from build123d import *

# Parameters (mm, degrees)
SKETCH_1_W          = 71.7
SKETCH_1_H          = 30.5
EXTRUDE_1_DEPTH     = 25
SHELL_1_T           = -3
CUT_EXTRUDE_1_REACH = 48.29
SKETCH_2_W          = 30
SKETCH_2_H          = 10
SKETCH_3_W          = 9
SKETCH_3_H          = 9
EXTRUDE_2_DEPTH     = 10
SKETCH_4_R          = 4.924428901
CUT_EXTRUDE_2_DEPTH = 72.41207881
FILLET_1_R          = 0.2
EXTRUDE_3_DEPTH     = 9
FILLET_2_R          = 0.2
FILLET_3_R          = 0.5
MIRROR_START        = 15.5
MIRROR_2_DEPTH      = 9
FILLET_5_R          = 0.5
FILLET_6_R          = 0.5


# Read off the part's stored shape, not the designer's step: 镜向2
with BuildPart() as part:
    # 草图1 → 凸台-拉伸1 (new body)
    with BuildSketch(Plane.XY):
        Rectangle(SKETCH_1_W, SKETCH_1_H)
    extrude(amount=EXTRUDE_1_DEPTH)

    # 抽壳1
    shell_1_openings = [part.faces().sort_by_distance(p)[0] for p in [
        (35.85, 0, 12.5),
    ]]
    offset(amount=SHELL_1_T, openings=shell_1_openings, kind=Kind.INTERSECTION)

    # 草图2 → 切除-拉伸1 (cut, up to next)
    with BuildSketch(Plane(origin=(0, 0, 0), x_dir=(-1, 0, 0), z_dir=(0, 0, -1)), mode=Mode.PRIVATE) as cut_extrude_1_sk1:
        with Locations((17.35, -6.95)):
            Rectangle(SKETCH_2_W, SKETCH_2_H)
    cut_extrude_1_tool1 = extrude(cut_extrude_1_sk1.sketch, amount=-CUT_EXTRUDE_1_REACH, mode=Mode.PRIVATE) & part.part
    add(cut_extrude_1_tool1.solids().sort_by_distance((-17.35, -6.95, 0))[0], mode=Mode.SUBTRACT)

    # 草图3 → 凸台-拉伸2 (add)
    with BuildSketch(Plane.XY.offset(25)):
        with Locations((-20, 0)):
            Rectangle(SKETCH_3_W, SKETCH_3_H)
        with Locations((20, 0)):
            Rectangle(SKETCH_3_W, SKETCH_3_H)
    extrude(amount=EXTRUDE_2_DEPTH)

    # 草图4 → 切除-拉伸2 (cut, through all)
    with BuildSketch(Plane.ZY.offset(24.5)):
        with Locations((37, 0)):
            Circle(SKETCH_4_R)
    extrude(amount=-CUT_EXTRUDE_2_DEPTH, mode=Mode.SUBTRACT)

    # 圆角1
    fillet_1_edges = [part.edges().sort_by_distance(p)[0] for p in [
        (-20, 4.5, 35),
        (-20, -4.5, 35),
        (20, 4.5, 35),
        (20, -4.5, 35),
    ]]
    fillet(fillet_1_edges, radius=FILLET_1_R)

    # 草图5 → 凸台-拉伸3 (add)
    with BuildSketch(Plane.ZY.offset(24.5)):
        Polygon((34.212569003, 4.5), (32.769193331, 7), (30.446869021, 7), (30.446869021, 6), (32.191843061, 6), (33.057868465, 4.5), align=None)
        Polygon((32.769193331, -7), (30.446869021, -7), (30.446869021, -6), (32.191843061, -6), (33.057868465, -4.5), (34.212569003, -4.5), align=None)
    extrude(amount=-EXTRUDE_3_DEPTH)

    # 圆角2
    fillet_2_edges = [part.edges().sort_by_distance(p)[0] for p in [
        (-20, 6, 32.191843061),
        (-20, 6, 30.446869021),
        (-20, 7, 30.446869021),
        (-20, 7, 32.769193331),
        (-20, -7, 32.769193331),
        (-20, -7, 30.446869021),
        (-20, -6, 30.446869021),
        (-20, -6, 32.191843061),
    ]]
    fillet(fillet_2_edges, radius=FILLET_2_R)

    # 圆角3
    fillet_3_edges = [part.edges().sort_by_distance(p)[0] for p in [
        (-20, 4.5, 33.057868465),
        (-20, -4.5, 33.057868465),
    ]]
    fillet(fillet_3_edges, radius=FILLET_3_R)

    # 镜向2 outline → 镜向2 (add)
    with BuildSketch(Plane.YZ.offset(MIRROR_START)):
        with BuildLine():
            Line((5.25, 32.624855763), (5.9, 32.249578088))
            ThreePointArc((5.9, 32.249578088), (5.973205081, 32.176373007), (6, 32.076373007))
            Line((6, 32.076373007), (6, 30.646869021))
            ThreePointArc((6, 30.646869021), (6.058578644, 30.505447665), (6.2, 30.446869021))
            Line((6.2, 30.446869021), (6.8, 30.446869021))
            ThreePointArc((6.8, 30.446869021), (6.941421356, 30.505447665), (7, 30.646869021))
            Line((7, 30.646869021), (7, 32.653723277))
            ThreePointArc((7, 32.653723277), (6.973205081, 32.753723277), (6.9, 32.826928357))
            Line((6.9, 32.826928357), (4.5, 34.212569003))
            Line((4.5, 34.212569003), (4.5, 32.191843061))
            ThreePointArc((4.5, 32.191843061), (4.75, 32.624855763), (5.25, 32.624855763))
        make_face()
        with BuildLine():
            Line((-6.8, 30.446869021), (-6.2, 30.446869021))
            ThreePointArc((-6.2, 30.446869021), (-6.058578644, 30.505447665), (-6, 30.646869021))
            Line((-6, 30.646869021), (-6, 32.076373007))
            ThreePointArc((-6, 32.076373007), (-5.973205081, 32.176373007), (-5.9, 32.249578088))
            Line((-5.9, 32.249578088), (-5.25, 32.624855763))
            ThreePointArc((-5.25, 32.624855763), (-4.75, 32.624855763), (-4.5, 32.191843061))
            Line((-4.5, 32.191843061), (-4.5, 34.212569003))
            Line((-4.5, 34.212569003), (-6.9, 32.826928357))
            ThreePointArc((-6.9, 32.826928357), (-6.973205081, 32.753723277), (-7, 32.653723277))
            Line((-7, 32.653723277), (-7, 30.646869021))
            ThreePointArc((-7, 30.646869021), (-6.941421356, 30.505447665), (-6.8, 30.446869021))
        make_face()
    extrude(amount=MIRROR_2_DEPTH)

    # 圆角5
    fillet_5_edges = [part.edges().sort_by_distance(p)[0] for p in [
        (-15.5, 0, 25),
        (-20, 4.5, 25),
        (-24.5, 0, 25),
        (-20, -4.5, 25),
    ]]
    fillet(fillet_5_edges, radius=FILLET_5_R)

    # 圆角6
    fillet_6_edges = [part.edges().sort_by_distance(p)[0] for p in [
        (24.5, 0, 25),
        (20, 4.5, 25),
        (15.5, 0, 25),
        (20, -4.5, 25),
    ]]
    fillet(fillet_6_edges, radius=FILLET_6_R)


solid = part.part
Design review of the part built by this model. Coordinates are the model's own, in mm. A direction names the side the tool comes from. Round coordinates to 2 decimals unless told otherwise and drop trailing zeros. Write each loop counter-clockwise with the first axis right and the second up, starting at its lowest first coordinate (ties: lowest second). Pieces come first, ordered by that corner, then holes. Notation, with made-up numbers: M -27,-35 L 24,-35 A24 cw 24,-22 Z; hole C -23.75,6.25 d10. An arc over 180 degrees is marked long. One line per item, written item: value. Start each with the question number.
1. Clearance check with flat-ended pins moving along their axes: P1, Ø2, axis at x = 20, z = 31.5, coming from the -Y side; P2, Ø2, axis at x = 18, z = 27.5, coming from the +Y side; P3, Ø3.5, axis at x = -19.5, z = 28.5, coming from the -Y side. State where each tip first meets the part, or that it passes through.
2. To check wall thickness, follow probe 1 along Z at (x, y) = (9, -6); probe 2 along Y at (x, z) = (17, 7.5); probe 3 along Y at (x, z) = (-20.5, 26.5). State the ranges of each line that lie inside material, in increasing order. Write a range as from..to.
3. For faces 5 (the face through (20, 7, 32)), 6 (the face through (-24.5, 0, 30)), 7 (the face through (1, 0, 22)), 8 (the face through (-32.35, -7, 1)), 9 (the face through (20, 6, 31)), list the 3-axis set-ups (+Z, -Z, +X, -X, +Y, -Y) from which the entire face can be reached by the end or side of a thin tool; tool diameter is ignored.
4. Take a section at B-B on x = 3. State the section outline as (y, z) points, then the cut area to 3 significant figures.
5. Take a section at D-D on z = 16. State the section outline as (x, y) points, then the cut area to 3 significant figures.
6. Take a section at C-C on y = 11. State the section outline as (x, z) points, then the cut area to 3 significant figures.
7. Draft analysis for pull direction X (two halves, no side actions). For faces 1 (the face through (-15.5, 0, 30)), 2 (the face through (-20, -4.5, 29)), 3 (the face through (15.5, 0, 30)), 4 (the face through (24.5, 0, 30)), state which applies: pulls with the +X half, pulls with the -X half, needs draft (parallel to the pull), parting line crosses it, or undercut.
8. Take a section at A-A on z = 29. State the section outline as (x, y) points, then the cut area to 3 significant figures.
Computed:
1. P1: stops at y = -7
1. P2: stops at y = 4.5
1. P3: stops at y = -4.5
2. probe 1: z = 0..3, 22..25
2. probe 2: y = -15.25..-12.25, 12.25..15.25
2. probe 3: y = -4.5..4.5
3. face 5: +Z, +X, -X, +Y
3. face 6: +Z, -X, +Y, -Y
3. face 7: +X
3. face 8: -Z
3. face 9: +X, -X
4. outline: M -15.25,0 L 15.25,0 L 15.25,25 L -15.25,25 Z; hole M -12.25,3 L 12.25,3 L 12.25,22 L -12.25,22 Z
4. area: 297 mm²
5. outline: M -35.85,-15.25 L 35.85,-15.25 L 35.85,-12.25 L -32.85,-12.25 L -32.85,12.25 L 35.85,12.25 L 35.85,15.25 L -35.85,15.25 Z
5. area: 504 mm²
6. outline: M -35.85,0 L 35.85,0 L 35.85,3 L -32.85,3 L -32.85,22 L 35.85,22 L 35.85,25 L -35.85,25 Z
6. area: 487 mm²
7. face 1: undercut
7. face 2: needs draft
7. face 3: undercut
7. face 4: pulls with the +X half
8. outline: M -24.5,-4.5 L -15.5,-4.5 L -15.5,4.5 L -24.5,4.5 Z; M 15.5,-4.5 L 24.5,-4.5 L 24.5,4.5 L 15.5,4.5 Z
8. area: 162 mm²
